```python
from build123d import *

# Parameters (mm, degrees)
CHANFREIN1_SIZE         = 0.5
ENL_V_MAT_EXTRU_1_DEPTH = 2.3


with BuildPart() as part:
    # Esquisse1 → Révolution1 (revolve)
    with BuildSketch(Plane.XY):
        Polygon((0, 0), (0, 5), (0.5, 5), (3, 2.5), (10, 2.5), (10, 0), align=None)
    revolve(axis=Axis((10, 0, 0), (-1, 0, 0)))

    # Chanfrein1
    chanfrein1_edges = [part.edges().sort_by_distance(p)[0] for p in [
        (10, -2.5, 0),
    ]]
    chamfer(chanfrein1_edges, length=CHANFREIN1_SIZE)

    # Esquisse2 → Enlèv. mat.-Extru.1 (cut)
    with BuildSketch(Plane.ZY):
        Polygon((0, 1.732050808), (-1.5, 0.866025404), (-1.5, -0.866025404), (0, -1.732050808), (1.5, -0.866025404), (1.5, 0.866025404), align=None)
    extrude(amount=-ENL_V_MAT_EXTRU_1_DEPTH, mode=Mode.SUBTRACT)


solid = part.part
```
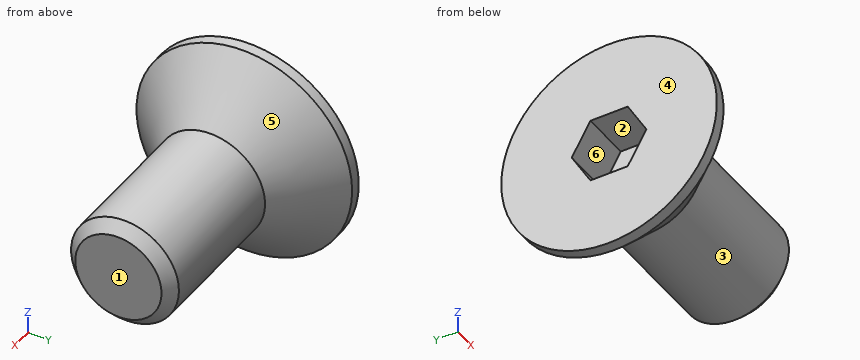
Geometry check sheet. Reference: the model listing, model coordinates, mm. Face numbers are marked on the shaded views. A direction names the side the tool comes from. Round coordinates to 2 decimals unless told otherwise and drop trailing zeros. Order: outer loops, then holes, each group sorted by start corner. A loop starts at its lowest first (then second) coordinate and runs counter-clockwise, first axis right, second up. Notation, with made-up numbers: M 58,89 L 65,89 A20 cw 65,95 Z; hole C 72,75.25 d3. An arc over 180 degrees is marked long. Write item = value, one per line.
Q1. Set-up check for the marked faces 1, 2 and 3: record each of +Z, -Z, +X, -X, +Y, -Y from which the full face is reachable in a straight line by a thin tool's end or side.
Answer block:
face_1 = +Z, -Z, +X, +Y, -Y
face_2 = -X
face_3 = +X
Q2. Scan lines: line 1 (X direction, y = -0.25, z = -0.5); line 2 (Z direction, x = 6.5, y = -1.5). Record each from-to range of solid material in increasing order.
Answer block:
line_1 = 2.3 to 10
line_2 = -2 to 2
Q3. Section check C-C (x = 4). Enter the section's corners in (y, z).
Answer block:
outline = C 0,0 d5
Q4. Depth check by flat-ended pin: pin 1 Ø1.5 at (x, y) = (9, -0.5) entering from -Z; pin 2 Ø3 at (x, z) = (8, -1.5) entering from +Y; pin 3 Ø0.9 at (y, z) = (0.5, 0.5) entering from -X. Enter the tip coordinate at first touch or a pass-through.
Answer block:
pin_1 = -2.5
pin_2 = 2.5
pin_3 = 2.3
Q5. Section check A-A (x = 1.25). Enter the section's corners in (y, z), plus the area to 3 significant figures.
Answer block:
outline = C 0,0 d8.5; hole M -1.73,0 L -0.87,-1.5 L 0.87,-1.5 L 1.73,0 L 0.87,1.5 L -0.87,1.5 Z
area = 49.0 mm^2
Q6. Section check B-B (y = 0). Enter the section's corners in (x, z), plus the area to 3 significant figures.
Answer block:
outline = M 0,-5 L 0.5,-5 L 3,-2.5 L 9.5,-2.5 L 10,-2 L 10,2 L 9.5,2.5 L 3,2.5 L 0.5,5 L 0,5 L 0,1.5 L 2.3,1.5 L 2.3,-1.5 L 0,-1.5 Z
area = 51.6 mm^2
Q7. Release check for a two-part mould opening along Z. For the marked faces 4, 5 and 6 record: released by +Z, released by -Z, zero draft, split by the parting line, or undercut.
Answer block:
face_4 = zero draft
face_5 = split by the parting line
face_6 = undercut
